Autodesk Inventor part; units mm, degrees
ref_plane "YZ Plane" through (0, 0, 0) normal (1, 0, 0) x (0, 1, 0)
ref_plane "XZ Plane" through (0, 0, 0) normal (0, 1, 0) x (-1, 0, 0)
ref_plane "XY Plane" through (0, 0, 0) normal (0, 0, 1) x (1, 0, 0)
sketch "Skizze1" plane through (0, 0, 0) normal (0, 1, 0) x (-1, 0, 0)
  circle A0 centre (0, 0) radius 2.6
  circle A1 centre (0, 0) radius 5
  line L0 (5, 0) -> (-5, 0)
  line L1 (-5, 0) -> (-5, -60)
  line L2 (-5, -60) -> (5, -60)
  line L3 (5, -60) -> (5, 0)
  circle A2 centre (0, -55) radius 5
  point P0 (-5, -55)
  point P1 (5, -55)
  dimension "d1" = 10
  dimension "d0" = 5.2
  dimension "d2" = 60
extrude "Extrusion1" add sketch "Skizze1" along normal blind 1 contours L0 A0 | L0 A1 A0 | A0 L0 A1 | A0 L0 | L3 A2 L1 A1 | A2
sketch "Skizze2" plane through (0, 1, 0) normal (0, 1, 0) x (1, 0, 0)
  circle A0 centre (0, 0) radius 2.575
  line L0 (-5, 55) -> (-5, 0)
  circle A1 centre (0, 0) radius 5
  dimension "d5" = 5.15
extrude "Extrusion2" add sketch "Skizze2" along normal blind 2.5
sketch "Skizze3" plane through (0, 1, 0) normal (0, 1, 0) x (1, 0, 0)
  circle A0 centre (0, 0) radius 1.5
  dimension "d8" = 3
extrude "Extrusion3" cut sketch "Skizze3" against normal blind 2.5
sketch "Skizze5" plane through (0, 1, 0) normal (0, 1, 0) x (1, 0, 0)
  arc A0 (5, 55) -> (-5, 55) centre (0, 55) ccw
  line L0 (5, 20) -> (-5, 20)
  line L1 (-5, 20) -> (-5, 55)
  line L2 (-5, 55) -> (5, 55)
  line L3 (5, 55) -> (5, 20)
  arc A1 (5, 55) -> (-5, 55) centre (0, 55) ccw
  point P0 (0, 0)
extrude "Extrusion4" add sketch "Skizze5" along normal blind 3
sketch "Skizze6" plane through (-5, 1, -20) normal (0, 0, 1) x (1, 0, 0)
  line L0 (0, 0) -> (0, 3)
  line L1 (0, 3) -> (0, 0)
  line L2 (10, 0) -> (0, 0)
  line L3 (0, 0) -> (10, 0)
  line L4 (0, 3) -> (10, 3)
  line L5 (10, 0) -> (0, 3)
  line L6 (0, -1) -> (0, 3)
  line L7 (0, 3) -> (10, 3)
  line L8 (10, -1) -> (10, 3)
  line L9 (10, 3) -> (10, 0)
  point P0 (5, -1)
extrude "Extrusion5" cut sketch "Skizze6" against normal blind 47 contours L4 L8 L5
fillet "Rundung1" radius 1.25 2 edges at (0, 2.5, -20) (-5, 2.5, -20)
equation "\"Biegeradius\" = Stärke"
equation "\"BreiteBiegungsfreistellung\" = Stärke"
equation "\"TiefeBiegungsfreistellung\" = 0.5 * Stärke"
equation "\"GrößeEckenfreistellung\" = 4 * Stärke"
equation "\"MinimalRest\" = 2 * Stärke"
equation "\"Übergangsradius\" = Biegeradius"
equation "\"JacobiRadiusGröße\" = Biegeradius"
equation "\"Abstandsgröße\" = Stärke"
properties part number "Pbj5"
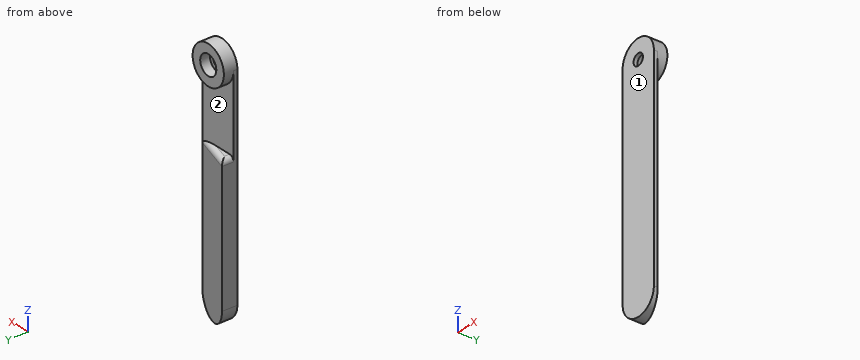
Check sheet for the modelled part. Datum: model origin and axes. Units: mm. Face numbers are marked on the shaded views. Coordinates: 2 decimals unless noted, no trailing zeros. Loops run counter-clockwise (first coordinate to the right, second up) from the corner with the lowest first, then second, coordinate; pieces in that order, holes last. Notation, with made-up numbers: (-1, 47) -> (45, 47) arc R31 ccw to (45, 71) -> close; hole circle Ø8 at (7, 86.25). An arc over 180 degrees is marked (long way). Write item = value, one per line. Start each with the question number.
1. Depth check by flat-ended pin: P1, Ø2.5, axis at x = 0, z = 0, coming from the -Y side; P2, Ø4, axis at x = 3, z = -23, coming from the +Y side; P3, Ø1, axis at x = -3.5, y = 1, coming from the +Z side; P4, Ø3, axis at x = -2, z = -5.5, coming from the +Y side. Enter the tip coordinate at first touch or a pass-through.
2. Section check B-B on z = -29. Record the cut outline in (x, y).
3. Section check A-A on y = 2.85. Give the number of separate pieces and of enclosed holes in the cut face, then the cut area to 3 significant figures.
4. Material ranges on line 1 (X direction, y = 0.45, z = 0); line 2 (Z direction, x = 0, y = 1.6) (3 decimals); line 3 (X direction, y = 2, z = 0) (3 decimals), recorded low to high.
5. Draft check along Z on the marked faces 1 and 2. Enter one of: released by +Z, released by -Z, zero draft, split by the parting line, or undercut.
Responses:
q1.P1 = through
q1.P2 = 2.2
q1.P3 = 4
q1.P4 = 3.5
q2.outline = (-5, 0) -> (5, 0) -> (5, 1) -> (-5, 4) -> close
q3.separate_pieces = 2
q3.enclosed_holes = 1
q3.area = 204 mm2
q4.line_1 = -5 to -1.5, 1.5 to 5
q4.line_2 = -60 to -20.062, -5 to -2.575, 2.575 to 5
q4.line_3 = -5 to -2.575, 2.575 to 5
q5.face_1 = zero draft
q5.face_2 = undercut
